Print and shaded views of the part. All mm, measured from the part's lowest x, y and z. Give positions to 0.01 mm unless a question says otherwise; leave off trailing zeros. Loops run counter-clockwise (first coordinate to the right, second up) from the corner with the lowest first, then second, coordinate; pieces in that order, holes last. Notation, with made-up numbers: (85.5, 80) -> (132.5, 80) arc R27 cw to (132.5, 117) -> close; hole circle Ø5 at (69.25, 29). An arc over 180 degrees is marked (long way). Answer as a JSON object with one key per item and string values. Group by question number.
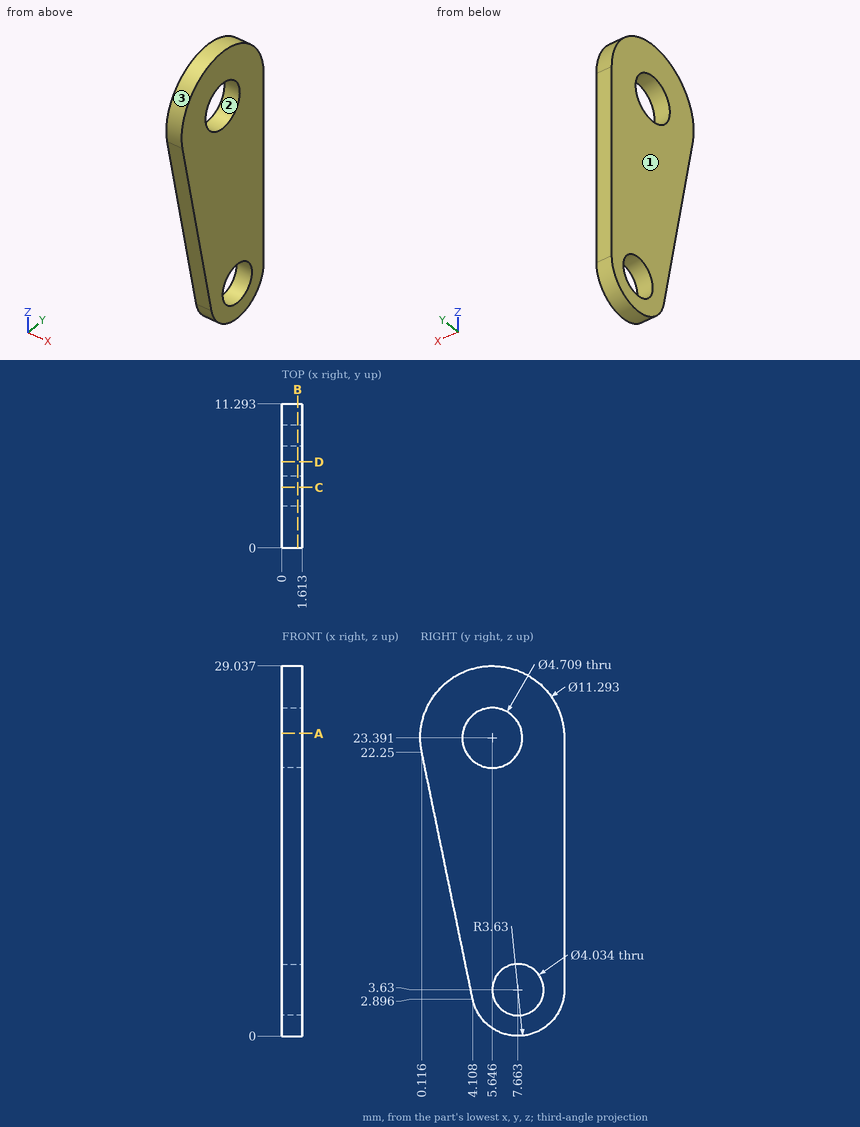
(1) Saw through at A-A on z = 23.75. List the corners of the cut face in (x, y).
(2) Saw through at D-D on y = 6.75. List the corners of the cut face in (x, z).
(3) Saw through at C-C on y = 4.75. List the corners of the cut face in (x, z) (1 decimal).
(4) Probe line 1 along Z through (x, y) = (1.3, 6) (1 decimal); line 2 along Z through (x, y) = (1, 6.25) (1 decimal); line 3 along Y through (x, z) = (0.35, 8.75). List the from-to ranges inside material, lowest first. Write a range as [from, to].
(5) Pull direction Y, two halves, no side cores. Call the marked faces 1, 2 and 3: pulls with the +Y half, pulls with the -Y half, needs draft (parallel to the pull), parting line crosses it, or undercut.
(6) Saw through at B-B on x = 1.25. Give the number of separate pieces and of enclosed holes in the cut face, plus the area to 3 significant figures.
Calculated:
{
 "1": {"outline": "(0, 0.01) -> (1.61, 0.01) -> (1.61, 3.32) -> (0, 3.32) -> close; (0, 7.97) -> (1.61, 7.97) -> (1.61, 11.28) -> (0, 11.28) -> close"},
 "2": {"outline": "(0, 0.12) -> (1.61, 0.12) -> (1.61, 1.83) -> (0, 1.83) -> close; (0, 5.43) -> (1.61, 5.43) -> (1.61, 21.31) -> (0, 21.31) -> close; (0, 25.47) -> (1.61, 25.47) -> (1.61, 28.93) -> (0, 28.93) -> close"},
 "3": {"outline": "(0, 1.5) -> (1.6, 1.5) -> (1.6, 21.2) -> (0, 21.2) -> close; (0, 25.6) -> (1.6, 25.6) -> (1.6, 29) -> (0, 29) -> close"},
 "4": {"line 1": "z = [0.4, 2.5], [4.8, 21.1], [25.7, 29]", "line 2": "z = [0.3, 2.2], [5.1, 21.1], [25.7, 29]", "line 3": "y = [2.9, 11.29]"},
 "5": {"face 1": "needs draft", "face 2": "undercut", "face 3": "parting line crosses it"},
 "6": {"separate pieces": "1", "enclosed holes": "2", "area": "226 mm^2"}
}
